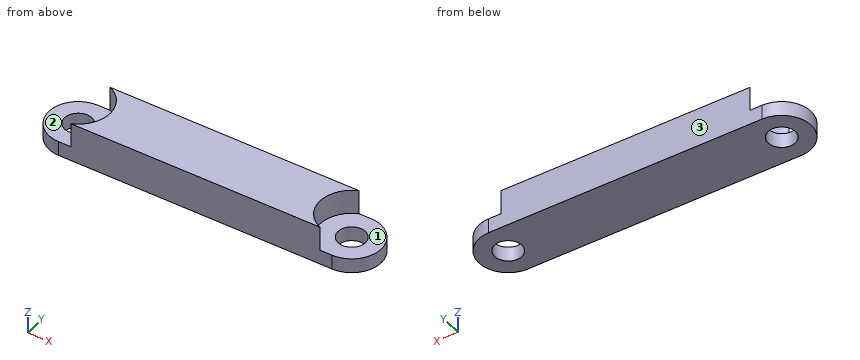
Autodesk Inventor part; units mm, degrees
ref_plane "YZ Plane" through (0, 0, 0) normal (1, 0, 0) x (0, 1, 0)
ref_plane "XZ Plane" through (0, 0, 0) normal (0, 1, 0) x (-1, 0, 0)
ref_plane "XY Plane" through (0, 0, 0) normal (0, 0, 1) x (1, 0, 0)
ref_plane "Arbeitsebene1" through (0, 0, 0) normal (0, 0, 1) x (1, 0, 0)
sketch "Skizze1" plane through (0, 0, 0) normal (0, 0, 1) x (1, 0, 0)
  circle A0 centre (17.5021, -9.9999) radius 1.45
  circle A1 centre (-17.4978, -9.9998) radius 1.45
  circle A2 centre (-17.4979, 10.0001) radius 1.45
  circle A3 centre (17.5021, 10.0001) radius 1.45
  arc A4 (-9.5, 21.063) -> (-12.4584, 22.8184) centre (-11.5, 21.063) ccw
  arc A5 (-12.4584, 22.8184) -> (12.4584, 22.8184) centre (0, 0) ccw
  arc A6 (12.4584, 22.8184) -> (9.5, 21.063) centre (11.5, 21.063) ccw
  line L0 (9.5, 21.063) -> (9.5, 17.6304)
  line L1 (9.5, 17.6304) -> (14, 17.6304)
  arc A7 (14, 10.6304) -> (14, 17.6304) centre (14, 14.1304) ccw
  line L2 (14, 10.6304) -> (9.5, 10.6304)
  line L3 (9.5, 10.6304) -> (9.5, -9)
  line L4 (9.5, -9) -> (-9.5, -9)
  line L5 (-9.5, -9) -> (-9.5, 10.6304)
  line L6 (-9.5, 10.6304) -> (-14, 10.6304)
  arc A8 (-14, 17.6304) -> (-14, 10.6304) centre (-14, 14.1304) ccw
  line L7 (-14, 17.6304) -> (-9.5, 17.6304)
  line L8 (-9.5, 17.6304) -> (-9.5, 21.063)
  circle A9 centre (-14, 14.1304) radius 1.4
  circle A10 centre (14, 14.1304) radius 1.4
  line L9 (-14, 14.1304) -> (14, 14.1304) construction
  line L10 (-14, 11.1304) -> (14, 11.1304)
  line L11 (14, 17.1304) -> (-14, 17.1304)
  arc A11 (-14, 17.1304) -> (-14, 11.1304) centre (-14, 14.1304) ccw
  arc A12 (14, 11.1304) -> (14, 17.1304) centre (14, 14.1304) ccw
  point P0 (0, 14.1304)
  dimension "d0" = 6
extrude "Extrusion1" add sketch "Skizze1" against normal blind 4 contours A11 L11 A12 L10
sketch "Skizze2" plane through (0, 0, 0) normal (0, 0, 1) x (1, 0, 0)
  arc A0 (14, 11.1304) -> (14, 17.1304) centre (14, 14.1304) ccw
  line L0 (14, 17.1304) -> (-14, 17.1304)
  arc A1 (-14, 17.1304) -> (-14, 11.1304) centre (-14, 14.1304) ccw
  line L1 (-14, 11.1304) -> (14, 11.1304)
  circle A2 centre (14, 14.1304) radius 1.4
  circle A3 centre (-14, 14.1304) radius 1.4
  point P0 (0, 0)
hole "Bohrung1" at (-14, 14.1304, 0) at (14, 14.1304, 0) direction (0, 0, -1) diameter 2.8 depth 7 tip angle 118 counterbore diameter 6.5 counterbore depth 2.5
sketch "Skizze3" plane through (-14, 17.1304, -4) normal (0, 1, 0) x (1, 0, 0)
  line L0 (1.25, -1.5) -> (1.25, -4)
  line L1 (26.75, -4) -> (1.25, -4)
  line L2 (26.75, -4) -> (26.75, -1.5)
  line L3 (26.75, -1.5) -> (28, -1.5)
  line L4 (28, -1.5) -> (28, 0)
  line L5 (0, 0) -> (28, 0)
  line L6 (0, -1.5) -> (0, 0)
  line L7 (0, -1.5) -> (1.25, -1.5)
  line L8 (-22.3971, 2) -> (50.3971, 2)
  circle A0 centre (14, 2) radius 2
  point P0 (14, -4)
properties part number "Cableholder_Ikealamp"
Here's how the part is built. I have some questions about the finished solid (model axes, mm). Face numbers are marked on the shaded views. A direction names the side the tool comes from. Coordinates: 2 decimals unless noted, no trailing zeros. Order: outer loops, then holes, each group sorted by start corner. A loop starts at its lowest first (then second) coordinate and runs counter-clockwise, first axis right, second up. Notation, with made-up numbers: (33, -31.5) -> (81, -31.5) arc R22 ccw to (81, -2.5) -> close; hole circle Ø8 at (-16.5, 31.5). An arc over 180 degrees is marked (long way). Answer in a Markdown table with one row per item.
(1) I want a section at D-D on y = 14.75. List the corners of the cut face in (x, z) for me, then the cut area to 3 significant figures.
Answer key:
| item | result |
|---|---|
| outline | (-16.94, -4) -> (-15.26, -4) -> (-15.26, -2.5) -> (-16.94, -2.5) -> close; (-12.74, -4) -> (12.74, -4) -> (12.74, -2.5) -> (10.81, -2.5) -> (10.81, 0) -> (-10.81, 0) -> (-10.81, -2.5) -> (-12.74, -2.5) -> close; (15.26, -4) -> (16.94, -4) -> (16.94, -2.5) -> (15.26, -2.5) -> close |
| area | 97.3 mm^2 |
(2) I want a section at B-B on x = 13.5. List the corners of the cut face in (y, z) for me, then the cut area to 3 significant figures.
Answer key:
| item | result |
|---|---|
| outline | (11.13, -4) -> (12.82, -4) -> (12.82, -2.5) -> (11.13, -2.5) -> close; (15.44, -4) -> (17.13, -4) -> (17.13, -2.5) -> (15.44, -2.5) -> close |
| area | 5.08 mm^2 |
(3) Please list where these lines run through material, in increasing order: probe 1 along Y at (x, z) = (14, -3.15); probe 2 along X at (y, z) = (13.75, -3.8); probe 3 along X at (y, z) = (13.5, -2.75).
Answer key:
| item | result |
|---|---|
| probe 1 | 11.13 to 12.73, 15.53 to 17.13 |
| probe 2 | -16.98 to -15.35, -12.65 to 12.65, 15.35 to 16.98 |
| probe 3 | -16.93 to -15.25, -12.75 to 12.75, 15.25 to 16.93 |
(4) Will this pin go through, and if not, where does the flat tip stop? pin 1 Ø3.5 at (x, y) = (-14, 14.13) entering from +Z.
Answer key:
| item | result |
|---|---|
| pin 1 | z = -2.5 |
(5) On a 3-axis mill with a long thin cutter (end or side, diameter ignored), from which of +Z, -Z, +X, -X, +Y, -Y can I reach the whole of each face in a straight line? I mean the marked faces 1, 2 and 3. Say none if no direction works.
Answer key:
| item | result |
|---|---|
| face 1 | +Z, +X |
| face 2 | +Z, -X |
| face 3 | +Z, -Z, +X, -X, +Y |
(6) I want a section at C-C on z = -3.6. List the corners of the cut face in (x, y) for me, then the cut area to 3 significant figures.
Answer key:
| item | result |
|---|---|
| outline | (-14, 11.13) -> (14, 11.13) arc R3 ccw to (14, 17.13) -> (-14, 17.13) arc R3 ccw to start; hole circle Ø2.8 at (-14, 14.13); hole circle Ø2.8 at (14, 14.13) |
| area | 184 mm^2 |
(7) I want a section at A-A on y = 13.5. List the corners of the cut face in (x, z) for me.
Answer key:
| item | result |
|---|---|
| outline | (-16.93, -4) -> (-15.25, -4) -> (-15.25, -2.5) -> (-16.93, -2.5) -> close; (-12.75, -4) -> (12.75, -4) -> (12.75, -2.5) -> (10.81, -2.5) -> (10.81, 0) -> (-10.81, 0) -> (-10.81, -2.5) -> (-12.75, -2.5) -> close; (15.25, -4) -> (16.93, -4) -> (16.93, -2.5) -> (15.25, -2.5) -> close |
